Source: CAD feature listing. Evaluate the final solid. Frame: model axes, mm. Face numbers are marked on the shaded views. Coordinates: 2 decimals unless noted, no trailing zeros. Order: outer loops, then holes, each group sorted by start corner. A loop starts at its lowest first (then second) coordinate and runs counter-clockwise, first axis right, second up. Notation, with made-up numbers: (4.5, -38) -> (40.5, -38) arc R15 ccw to (40.5, -15) -> close; hole circle Ø10 at (-24.75, -5). An arc over 180 degrees is marked (long way). Put each result on its own line as item: value.
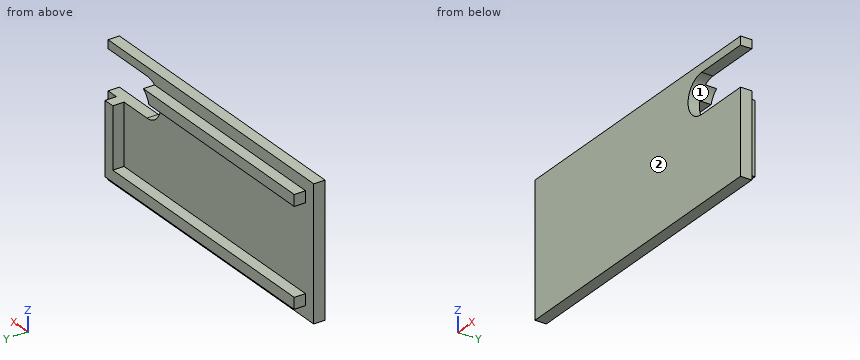
from build123d import *

# Parameters (mm, degrees)
SKETCH1_W           = 52.9
SKETCH1_H           = 23.3
BOSS_EXTRUDE1_DEPTH = 2
BOSS_EXTRUDE2_DEPTH = 2
CUT_EXTRUDE1_DEPTH  = 5


with BuildPart() as part:
    # Sketch1 → Boss-Extrude1 (new body)
    with BuildSketch(Plane(origin=(0, 0, 0), x_dir=(1, 0, 0), z_dir=(0, 1, 0))):
        with Locations((26.45, 11.65)):
            Rectangle(SKETCH1_W, SKETCH1_H)
    extrude(amount=BOSS_EXTRUDE1_DEPTH)

    # Sketch2 → Boss-Extrude2 (add)
    with BuildSketch(Plane(origin=(0, 2, 0), x_dir=(1, 0, 0), z_dir=(0, 1, 0))):
        Polygon((2.1, 21.2), (50.8, 21.2), (50.8, 2.1), (2.1, 2.1), (2.1, 4.1), (4.1, 4.1), (48.8, 4.1), (48.8, 19.2), (4.1, 19.2), (2.1, 19.2), align=None)
    extrude(amount=BOSS_EXTRUDE2_DEPTH)

    # Sketch3 → Cut-Extrude1 (cut, through all)
    with BuildSketch(Plane.XZ):
        with BuildLine():
            Line((42.9, -1.5), (53.235207038, -1.5))
            ThreePointArc((53.235207038, -1.5), (56.735207038, -5), (53.235207038, -8.5))
            Line((53.235207038, -8.5), (42.9, -8.5))
            ThreePointArc((42.9, -8.5), (39.4, -5), (42.9, -1.5))
        make_face()
    extrude(amount=-CUT_EXTRUDE1_DEPTH, mode=Mode.SUBTRACT)


solid = part.part
1. First-contact query: pin 1 (0.6 mm diameter, centred on x = 27.5, y = 3.5, fed in from -Z); pin 2 (1.6 mm diameter, centred on y = 3, z = -13.5, fed in from -X); pin 3 (1 mm diameter, centred on y = 3, z = -3, fed in from -X). Flat tips, straight axial feed; report the tip coordinate or a pass-through.
Numbers:
pin 1: stops at z = -21.2
pin 2: stops at x = 48.8
pin 3: stops at x = 2.1
2. Cut plane D-D on x = 25.5. Output: boundary loops of the cut face in (y, z), plus the area to 3 significant figures.
Numbers:
outline: (0, -23.3) -> (2, -23.3) -> (2, -21.2) -> (4, -21.2) -> (4, -19.2) -> (2, -19.2) -> (2, -4.1) -> (4, -4.1) -> (4, -2.1) -> (2, -2.1) -> (2, 0) -> (0, 0) -> close
area: 54.6 mm2
3. Cut plane A-A on x = 45. Output: boundary loops of the cut face in (y, z), plus the area to 3 significant figures.
Numbers:
outline: (0, -23.3) -> (2, -23.3) -> (2, -21.2) -> (4, -21.2) -> (4, -19.2) -> (2, -19.2) -> (2, -8.5) -> (0, -8.5) -> close; (0, -1.5) -> (2, -1.5) -> (2, 0) -> (0, 0) -> close
area: 36.6 mm2
4. Pull-direction query (Z, two-part tool) for the marked faces 1 and 2; classes: pulls with the +Z half, pulls with the -Z half, needs draft (parallel to the pull), parting line crosses it, or undercut.
Numbers:
face 1: undercut
face 2: needs draft
5. Ray query, line 1 along Z through (x, y) = (22, 3.7); line 2 along Y through (x, z) = (26, -9); line 3 along X through (y, z) = (2.45, -14). Return the intervals inside material, ascending.
Numbers:
line 1: z = -21.2 to -19.2, -4.1 to -2.1
line 2: y = 0 to 2
line 3: x = 48.8 to 50.8
6. Cut plane C-C on z = -9. Output: boundary loops of the cut face in (x, y), plus the area to 3 significant figures.
Numbers:
outline: (0, 0) -> (52.9, 0) -> (52.9, 2) -> (50.8, 2) -> (50.8, 4) -> (48.8, 4) -> (48.8, 2) -> (0, 2) -> close
area: 110 mm2
7. Cut plane B-B on y = 2.75. Output: boundary loops of the cut face in (x, z), plus the area to 3 significant figures.
Numbers:
outline: (2.1, -21.2) -> (50.8, -21.2) -> (50.8, -8.5) -> (48.8, -8.5) -> (48.8, -19.2) -> (2.1, -19.2) -> close; (2.1, -4.1) -> (39.52, -4.1) arc R3.5 cw to (40.94, -2.1) -> (2.1, -2.1) -> close
area: 195 mm2
